Could you check a few things on this model? Use its own coordinates, in mm. A direction names the side the tool comes from. Coordinates: 2 decimals unless noted, no trailing zeros. Order: outer loops, then holes, each group sorted by start corner. A loop starts at its lowest first (then second) coordinate and runs counter-clockwise, first axis right, second up. Notation, with made-up numbers: (4.25, 2) - (55.25, 2) arc R20 cw to (55.25, 6) - close; hole circle Ø2 at (7, -24). An arc over 180 degrees is marked (long way). One line per item, written item: value.
from build123d import *

# Parameters (mm, degrees)
SKIZZE1_W                       = 20
SKIZZE1_H                       = 9.5
AUFSATZ_LINEAR_AUSTRAGEN1_DEPTH = 6.4
AUFSATZ_LINEAR_AUSTRAGEN2_DEPTH = 13


with BuildPart() as part:
    # Skizze1 → Aufsatz-Linear austragen1 (new body)
    with BuildSketch(Plane(origin=(0, 0, 0), x_dir=(1, 0, 0), z_dir=(0, 1, 0))):
        Polygon((3.63728013, 8), (5.36271987, 8), (-8.27456026, 4.75), (-10, 4.75), align=None)
        Rectangle(SKIZZE1_W, SKIZZE1_H)
    extrude(amount=AUFSATZ_LINEAR_AUSTRAGEN1_DEPTH)

    # Skizze1_3 → Aufsatz-Linear austragen2 (add)
    with BuildSketch(Plane(origin=(0, 0, 0), x_dir=(1, 0, 0), z_dir=(0, 1, 0))):
        Polygon((3.63728013, 8), (0, 7.133173161), (1.72543974, 7.133173161), (5.36271987, 8), align=None)
    extrude(amount=AUFSATZ_LINEAR_AUSTRAGEN2_DEPTH)


solid = part.part
Item 1: If I drill on probe 1 along Y at (x, z) = (-1, -1.5); probe 2 along Z at (x, y) = (8.25, 4.5); probe 3 along Z at (x, y) = (-1.25, 2.5), over which ranges is the centre line in solid material (lowest first)?
Conclusion:
probe 1: 0 to 6.4
probe 2: -4.75 to 4.75
probe 3: -6.84 to -6.42, -4.75 to 4.75
Item 2: I want a section at C-C on z = -3.5. Please give me the cut outline in (x, y).
Conclusion:
outline: (-10, 0) - (10, 0) - (10, 6.4) - (-10, 6.4) - close
Item 3: I want a section at B-B on x = 1.25. Please give me the cut outline in (y, z), then the cut area to 3 significant figures.
Conclusion:
outline: (0, -7.43) - (13, -7.43) - (13, -7.13) - (6.4, -7.13) - (6.4, -7.02) - (0, -7.02) - close; (0, -4.75) - (6.4, -4.75) - (6.4, 4.75) - (0, 4.75) - close
area: 65.4 mm²
Item 4: I'm going to push flat-ended pins straight in: pin 1 Ø6 at (x, z) = (-3, -2.5) entering from +Y; pin 2 Ø1.9 at (x, y) = (0.5, 8.5) entering from +Z; pin 3 Ø2 at (y, z) = (9, -5.5) entering from +X; pin 4 Ø3 at (x, y) = (-3, 2.5) entering from -Z. Where does each tip first touch, or does it pass through?
Conclusion:
pin 1: y = 6.4
pin 2: z = -7.13
pin 3: through
pin 4: z = -6.78
Item 5: I want a section at A-A on y = 5.25. Please give me the cut outline in (x, z).
Conclusion:
outline: (-10, -4.75) - (3.64, -8) - (5.36, -8) - (-8.27, -4.75) - (10, -4.75) - (10, 4.75) - (-10, 4.75) - close
Item 6: I want a section at D-D on x = 8. Please give me the cut outline in (y, z), then the cut area to 3 significant figures.
Conclusion:
outline: (0, -4.75) - (6.4, -4.75) - (6.4, 4.75) - (0, 4.75) - close
area: 60.8 mm²
Item 7: For faces 1 (the face through (0, 6.4, 0)), 2 (the face through (4, 6, -8)), 3 (the face through (1, 3, -4.75)), which set-ups out of +Z, -Z, +X, -X, +Y, -Y let a thin tool reach every point of the face, with its end or its side?
Conclusion:
face 1: +Z, +X, -X, +Y
face 2: -Z, +X, -X, +Y, -Y
face 3: +X, +Y, -Y
